The figure shows three views and two pictorial views of one solid part (mm, origin at its lowest corner). Answer the questions. Round coordinates to 2 decimals unless told otherwise and drop trailing zeros. Order: outer loops, then holes, each group sorted by start corner. A loop starts at its lowest first (then second) coordinate and runs counter-clockwise, first axis right, second up. Notation, with made-up numbers: (42, 62) - (49, 62) arc R32 cw to (49, 96) - close; hole circle Ø1 at (-28, 54). An arc over 180 degrees is marked (long way). One line per item, written item: value. Start each with the question number.
1. Straight lines are drawn through the part: line 1 (Y direction, x = 205, z = 7) (3 decimals); line 2 (X direction, y = 116, z = 1.5); line 3 (Y direction, x = 160, z = 2.45). For each, find the intervals that lie inside material, in ascending order.
2. Section B-B, the plane z = 7 is taken. Count the separate pieces of the cut face and the enclosed holes in it, then the cut area to 3 significant figures.
3. Flat-ended cylindrical pins translate along their axes: P1, Ø18, axis at x = 115, y = 25, coming from the +Z side; P2, Ø19.5, axis at x = 31, y = 118.5, coming from the +Z side. Find the tip coordinate at first contact, or state that the pin passes through.
4. Section A-A, the plane x = 115 is taken. Give the vertices of the cut face in (y, z) (3 decimals).
5. Section C-C, the plane y = 39.5 is taken. Give the vertices of the cut face in (x, z), then the cut area to 3 significant figures.
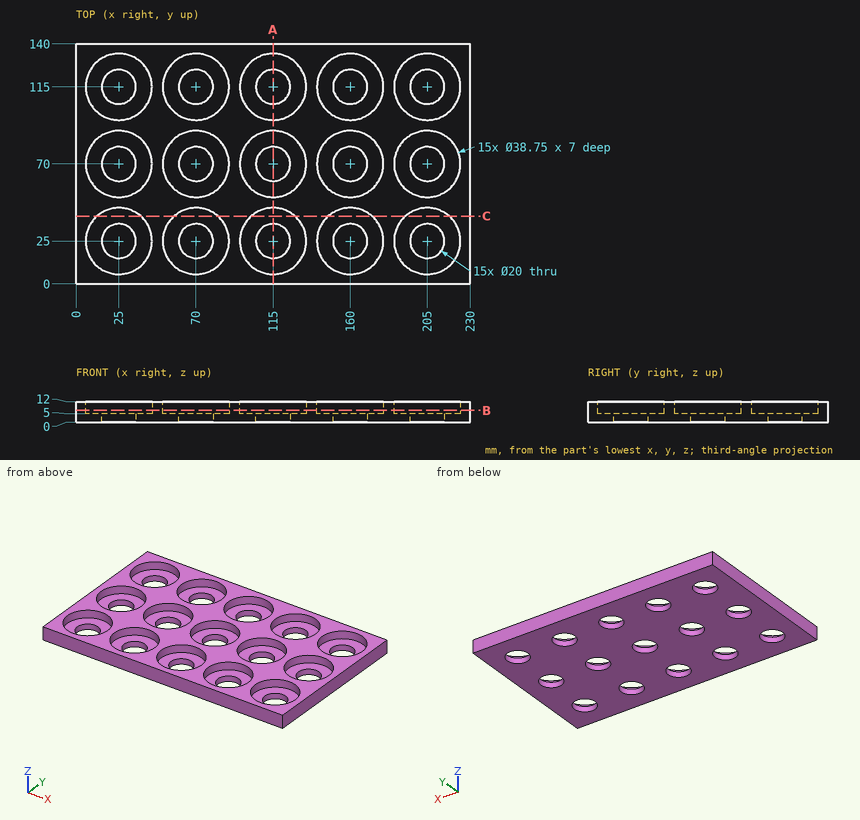
Answer list:
1. line 1: y = 0 to 5.625, 44.375 to 50.625, 89.375 to 95.625, 134.375 to 140
1. line 2: x = 0 to 15.05, 34.95 to 60.05, 79.95 to 105.05, 124.95 to 150.05, 169.95 to 195.05, 214.95 to 230
1. line 3: y = 0 to 15, 35 to 60, 80 to 105, 125 to 140
2. separate pieces: 1
2. enclosed holes: 15
2. area: 14,500 mm²
3. P1: passes through
3. P2: stops at z = 5
4. outline: (0, 0) - (15, 0) - (15, 5) - (5.625, 5) - (5.625, 12) - (0, 12) - close; (35, 0) - (60, 0) - (60, 5) - (50.625, 5) - (50.625, 12) - (44.375, 12) - (44.375, 5) - (35, 5) - close; (80, 0) - (105, 0) - (105, 5) - (95.625, 5) - (95.625, 12) - (89.375, 12) - (89.375, 5) - (80, 5) - close; (125, 0) - (140, 0) - (140, 12) - (134.375, 12) - (134.375, 5) - (125, 5) - close
5. outline: (0, 0) - (230, 0) - (230, 12) - (217.85, 12) - (217.85, 5) - (192.15, 5) - (192.15, 12) - (172.85, 12) - (172.85, 5) - (147.15, 5) - (147.15, 12) - (127.85, 12) - (127.85, 5) - (102.15, 5) - (102.15, 12) - (82.85, 12) - (82.85, 5) - (57.15, 5) - (57.15, 12) - (37.85, 12) - (37.85, 5) - (12.15, 5) - (12.15, 12) - (0, 12) - close
5. area: 1,860 mm²
